```python
from build123d import *

# Parameters (mm, degrees)
SKETCH1_W               = 120
SKETCH1_H               = 54
BOSS_EXTRUDE1_DEPTH     = 5.5
SKETCH2_W               = 120
SKETCH2_H               = 54
SKETCH2_W_2             = 116
SKETCH2_H_2             = 50
BOSS_EXTRUDE2_DEPTH     = 45
SKETCH3_W               = 9
SKETCH3_H               = 50
BOSS_EXTRUDE3_DEPTH     = 5
SKETCH4_R               = 1.65
CUT_EXTRUDE5_DEPTH      = 14
SKETCH5_W               = 10
SKETCH5_H               = 15
CUT_EXTRUDE7_DEPTH      = 139.416942605
FILLET1_R               = 0.7
FILLET2_R               = 0.7
FILLET3_R               = 0.7
FILLET4_R               = 0.7
FILLET5_R               = 0.7
FILLET6_R               = 0.7
FILLET7_R               = 0.7
FILLET8_R               = 0.7
CUT_EXTRUDE8_DEPTH      = 109.509763737
CUT_EXTRUDE8_DEPTH_BACK = 109.509763737


with BuildPart() as part:
    # Sketch1 → Boss-Extrude1 (new body)
    with BuildSketch(Plane.XY):
        with Locations((-20.747252747, 20)):
            Rectangle(SKETCH1_W, SKETCH1_H)
    extrude(amount=BOSS_EXTRUDE1_DEPTH)

    # Sketch2 → Boss-Extrude2 (add)
    with BuildSketch(Plane.XY.offset(5.5)):
        with Locations((-20.747252747, 20)):
            Rectangle(SKETCH2_W, SKETCH2_H)
        with Locations((-20.747252747, 20)):
            Rectangle(SKETCH2_W_2, SKETCH2_H_2, mode=Mode.SUBTRACT)
    extrude(amount=BOSS_EXTRUDE2_DEPTH)

    # Sketch3 → Boss-Extrude3 (add)
    with BuildSketch(Plane.XY.offset(5.5)):
        with Locations((-59.247252747, 20)):
            Rectangle(SKETCH3_W, SKETCH3_H)
        with Locations((-22.247252747, 20)):
            Rectangle(SKETCH3_W, SKETCH3_H)
        with Locations((14.752747253, 20)):
            Rectangle(SKETCH3_W, SKETCH3_H)
    extrude(amount=BOSS_EXTRUDE3_DEPTH)

    # Sketch4 → Cut-Extrude5 (cut)
    with BuildSketch(Plane.XY.offset(5.5)):
        with Locations((-4.74254548, 39.5)):
            Circle(SKETCH4_R)
        with Locations((-42.205415824, 39.5)):
            Circle(SKETCH4_R)
        with Locations((-72.673636324, 39.5)):
            Circle(SKETCH4_R)
        with Locations((29.282276635, 39.5)):
            Circle(SKETCH4_R)
    extrude(amount=-CUT_EXTRUDE5_DEPTH, mode=Mode.SUBTRACT)

    # Sketch5 → Cut-Extrude7 (cut, through all)
    with BuildSketch(Plane(origin=(39.252747253, 0, 0), x_dir=(0, 0, -1), z_dir=(1, 0, 0))):
        with Locations((-45.5, 20)):
            Rectangle(SKETCH5_W, SKETCH5_H)
    extrude(amount=-CUT_EXTRUDE7_DEPTH, mode=Mode.SUBTRACT)

    # Fillet1
    fillet1_edges = [part.edges().sort_by_distance(p)[0] for p in [
        (38.252747253, 12.5, 40.5),
    ]]
    fillet(fillet1_edges, radius=FILLET1_R)

    # Fillet2
    fillet2_edges = [part.edges().sort_by_distance(p)[0] for p in [
        (38.252747253, 27.5, 40.5),
    ]]
    fillet(fillet2_edges, radius=FILLET2_R)

    # Fillet3
    fillet3_edges = [part.edges().sort_by_distance(p)[0] for p in [
        (-79.747252747, 12.5, 40.5),
    ]]
    fillet(fillet3_edges, radius=FILLET3_R)

    # Fillet4
    fillet4_edges = [part.edges().sort_by_distance(p)[0] for p in [
        (-79.747252747, 27.5, 40.5),
    ]]
    fillet(fillet4_edges, radius=FILLET4_R)

    # Fillet5
    fillet5_edges = [part.edges().sort_by_distance(p)[0] for p in [
        (-79.747252747, 12.5, 50.5),
    ]]
    fillet(fillet5_edges, radius=FILLET5_R)

    # Fillet6
    fillet6_edges = [part.edges().sort_by_distance(p)[0] for p in [
        (-79.747252747, 27.5, 50.5),
    ]]
    fillet(fillet6_edges, radius=FILLET6_R)

    # Fillet7
    fillet7_edges = [part.edges().sort_by_distance(p)[0] for p in [
        (38.252747253, 12.5, 50.5),
    ]]
    fillet(fillet7_edges, radius=FILLET7_R)

    # Fillet8
    fillet8_edges = [part.edges().sort_by_distance(p)[0] for p in [
        (38.252747253, 27.5, 50.5),
    ]]
    fillet(fillet8_edges, radius=FILLET8_R)

    # Sketch6 → Cut-Extrude8 (cut, two sides: drawn at the far end of the back side and taken through both)
    with BuildSketch(Plane(origin=(0, -5, 0), x_dir=(1, 0, 0), z_dir=(0, 1, 0)).offset(-CUT_EXTRUDE8_DEPTH_BACK)):
        with BuildLine():
            Line((-49.247252747, -7), (-34.247252747, -7))
            ThreePointArc((-34.247252747, -7), (-32.747252747, -8.5), (-34.247252747, -10))
            Line((-34.247252747, -10), (-49.247252747, -10))
            ThreePointArc((-49.247252747, -10), (-50.747252747, -8.5), (-49.247252747, -7))
        make_face()
        with BuildLine():
            Line((-11.247252747, -7), (3.752747253, -7))
            ThreePointArc((3.752747253, -7), (5.252747253, -8.5), (3.752747253, -10))
            Line((3.752747253, -10), (-11.247252747, -10))
            ThreePointArc((-11.247252747, -10), (-12.747252747, -8.5), (-11.247252747, -7))
        make_face()
    extrude(amount=CUT_EXTRUDE8_DEPTH + CUT_EXTRUDE8_DEPTH_BACK, mode=Mode.SUBTRACT)


solid = part.part
```
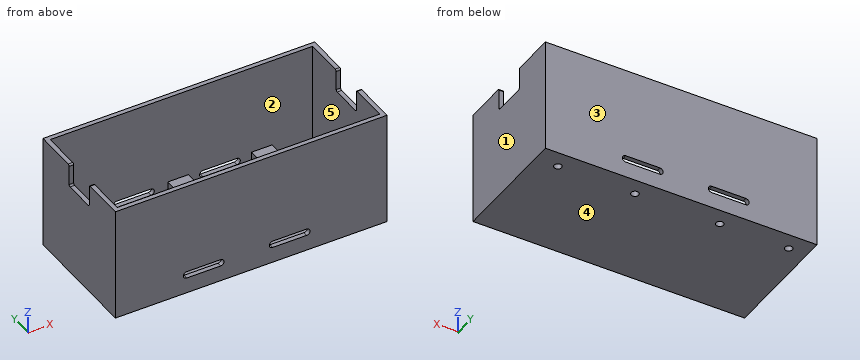
Model file for the job. Use its own axes, mm. Face numbers are marked on the shaded views. A direction names the side the tool comes from. Coordinates: 2 decimals unless noted, no trailing zeros. Loops run counter-clockwise (first coordinate to the right, second up) from the corner with the lowest first, then second, coordinate; pieces in that order, holes last. Notation, with made-up numbers: M 78,-27.75 L 103,-27.75 A20 ccw 103,-1.75 Z; hole C 78.25,87 d9. An arc over 180 degrees is marked long. Use CSV: the item, a comma, the result in double quotes. Start each with the question number.
1. Two-plate mould, pull along X, no slides. Class the marked faces 1, 2 and 3: pulls with the +X half, pulls with the -X half, needs draft (parallel to the pull), parting line crosses it, or undercut.
2. Band-saw the part on A-A, the plane z = 19. List the corners of the cut face in (x, y), then the cut area to 3 significant figures.
3. Band-saw the part on C-C, the plane x = -16.5. List the corners of the cut face in (y, z), then the cut area to 3 significant figures.
4. Band-saw the part on D-D, the plane z = 8.5. Give the number of separate pieces and of enclosed holes in the cut face, then the cut area to 3 significant figures.
5. Flat gauge pins, fed straight in: pin 1 (2 mm diameter, centred on x = 16.5, y = 34, fed in from +Z); pin 2 (9 mm diameter, centred on x = 25, y = 21.5, fed in from +Z). Where does each tip first touch, or does it go through?
6. Tool access for the marked faces 4 and 5: list every direction of +Z, -Z, +X, -X, +Y, -Y with a clear straight run to the whole face (end or side of a thin tool).
7. Band-saw the part on B-B, the plane y = 17.5. List the corners of the cut face in (x, z).
8. Probe probe 1 along X at (y, z) = (19, 9); probe 2 along X at (y, z) = (34.5, 34); probe 3 along Y at (x, z) = (12.5, 36.5). List the from-to ranges inside material, lowest first. Write a range as [from, to].
Entries:
1,face 1,"pulls with the +X half"
1,face 2,"undercut"
1,face 3,"needs draft"
2,outline,"M -80.75,-7 L 39.25,-7 L 39.25,47 L -80.75,47 Z; hole M -78.75,-5 L 37.25,-5 L 37.25,45 L -78.75,45 Z"
2,area,"680 mm2"
3,outline,"M -7,0 L 47,0 L 47,50.5 L 45,50.5 L 45,5.5 L -5,5.5 L -5,50.5 L -7,50.5 Z"
3,area,"477 mm2"
4,separate pieces,"3"
4,enclosed holes,"2"
4,area,"1,890 mm2"
5,pin 1,"stops at z = 10.5"
5,pin 2,"stops at z = 5.5"
6,face 4,"-Z, +X, -X, +Y, -Y"
6,face 5,"+Z"
7,outline,"M -80.75,0 L 39.25,0 L 39.25,40.5 L 37.25,40.5 L 37.25,5.5 L 19.25,5.5 L 19.25,10.5 L 10.25,10.5 L 10.25,5.5 L -17.75,5.5 L -17.75,10.5 L -26.75,10.5 L -26.75,5.5 L -54.75,5.5 L -54.75,10.5 L -63.75,10.5 L -63.75,5.5 L -78.75,5.5 L -78.75,40.5 L -80.75,40.5 Z"
8,probe 1,"x = [-80.75, -78.75], [-63.75, -54.75], [-26.75, -17.75], [10.25, 19.25], [37.25, 39.25]"
8,probe 2,"x = [-80.75, -78.75], [37.25, 39.25]"
8,probe 3,"y = [-7, -5], [45, 47]"
